from build123d import *
from build123d.topology import SkipClean

# Parameters (mm, degrees)
BOSS_EXTRUDE1_DEPTH  = 2
SKETCH12_R           = 25
BOSS_EXTRUDE2_DEPTH  = 8
CUT_EXTRUDE6_START   = -36
SKETCH17_R           = 10.33
CUT_EXTRUDE6_DEPTH   = 45.856111051
SKETCH25_R           = 30
BOSS_EXTRUDE3_DEPTH  = 5
CUT_EXTRUDE9_START   = -5
SKETCH26_R           = 10.33
CUT_EXTRUDE9_DEPTH   = 5
CUT_EXTRUDE10_DEPTH  = 45
FILLET3_R            = 1.5
MIRROR9_COPY_1_DEPTH = 45
FILLET3_OF_MIRROR9_R = 1.5
SKETCH29_R           = 10.33
CUT_EXTRUDE11_DEPTH  = 5


with BuildPart() as part:
    # Sketch3 → Boss-Extrude1 (new body)
    with BuildSketch(Plane(origin=(0, 0, 0), x_dir=(1, 0, 0), z_dir=(0, 1, 0))):
        Polygon((35.1, 0), (24.81944802, 24.81944802), (0, 35.1), (-24.81944802, 24.81944802), (-35.1, 0), (-24.81944802, -24.81944802), (0, -35.1), (24.81944802, -24.81944802), align=None)
    boss_extrude1 = extrude(amount=BOSS_EXTRUDE1_DEPTH)

    # Sketch12 → Boss-Extrude2 (add)
    with BuildSketch(Plane(origin=(0, 2, 0), x_dir=(1, 0, 0), z_dir=(0, 1, 0))):
        with Locations(Location((0, 0, 0), (0, 0, 270))):
            Circle(SKETCH12_R)
    boss_extrude2 = extrude(amount=BOSS_EXTRUDE2_DEPTH)

    # Sketch17 → Cut-Extrude6 (cut)
    with BuildSketch(Plane(origin=(0, 10, 0), x_dir=(1, 0, 0), z_dir=(0, 1, 0)).offset(CUT_EXTRUDE6_START)):
        with Locations(Location((0, 17, 0), (0, 0, 40.756206315))):
            Circle(SKETCH17_R)
    cut_extrude6 = extrude(amount=CUT_EXTRUDE6_DEPTH, mode=Mode.SUBTRACT)

    # Sketch25 → Boss-Extrude3 (add)
    with BuildSketch(Plane(origin=(0, 10, 0), x_dir=(1, 0, 0), z_dir=(0, 1, 0))):
        with Locations(Location((0, 0, 0), (0, 0, 270))):
            Circle(SKETCH25_R)
    boss_extrude3 = extrude(amount=BOSS_EXTRUDE3_DEPTH)

    # Sketch26 → Cut-Extrude9 (cut)
    with BuildSketch(Plane(origin=(0, 15, 0), x_dir=(1, 0, 0), z_dir=(0, 1, 0)).offset(CUT_EXTRUDE9_START)):
        with Locations(Location((0, 17, 0), (0, 0, 270))):
            Circle(SKETCH26_R)
    extrude(amount=CUT_EXTRUDE9_DEPTH, mode=Mode.SUBTRACT)

    # Sketch27 → Cut-Extrude10 (cut)
    with BuildSketch(Plane(origin=(0, 15, 0), x_dir=(1, 0, 0), z_dir=(0, 1, 0))):
        with BuildLine():
            Line((0, -20), (0, 4.5))
            ThreePointArc((0, 4.5), (-10.662403413, 8.877487957), (-21.5, 4.953746429))
            Line((-21.5, 4.953746429), (-21.5, -20))
            ThreePointArc((-21.5, -20), (-10.75, -24.149367106), (0, -20))
        make_face()
    cut_extrude10 = extrude(amount=-CUT_EXTRUDE10_DEPTH, mode=Mode.SUBTRACT)

    # Mirror8: Cut-Extrude10 across plane
    add(cut_extrude10.mirror(Plane.ZY), mode=Mode.SUBTRACT)

    # Fillet3
    fillet3_edges = [part.edges().sort_by_distance(p)[0] for p in [
        (12.40972401, 2, -29.95972401),
        (-12.40972401, 2, -29.95972401),
        (-29.95972401, 2, -12.40972401),
        (-29.95972401, 2, 12.40972401),
        (-12.40972401, 2, 29.95972401),
        (12.40972401, 2, 29.95972401),
        (29.95972401, 2, 12.40972401),
        (29.95972401, 2, -12.40972401),
    ]]
    fillet(fillet3_edges, radius=FILLET3_R)

    # Mirror9: Boss-Extrude1, Boss-Extrude2, Cut-Extrude6, Boss-Extrude3, Cut-Extrude10 across plane
    with SkipClean():  # the faces are left unmerged after this step: merging them gives an invalid solid
        add(boss_extrude1.mirror(Plane.ZX))
        add(boss_extrude2.mirror(Plane.ZX))
        add(cut_extrude6.mirror(Plane.ZX), mode=Mode.SUBTRACT)
        add(boss_extrude3.mirror(Plane.ZX))
        add(cut_extrude10.mirror(Plane.ZX), mode=Mode.SUBTRACT)

    # Mirror9 copy 1 sketch → Mirror9 copy 1 (cut)
    with SkipClean():  # the faces are left unmerged after this step: merging them gives an invalid solid
        with BuildSketch(Plane(origin=(0, -15, 0), x_dir=(-1, 0, 0), z_dir=(0, -1, 0))):
            with BuildLine():
                Line((0, -20), (0, 4.5))
                ThreePointArc((0, 4.5), (-10.662403413, 8.877487957), (-21.5, 4.953746429))
                Line((-21.5, 4.953746429), (-21.5, -20))
                ThreePointArc((-21.5, -20), (-10.75, -24.149367106), (0, -20))
            make_face()
        extrude(amount=-MIRROR9_COPY_1_DEPTH, mode=Mode.SUBTRACT)

    # Fillet3 of Mirror9
    fillet3_of_mirror9_edges = [part.edges().sort_by_distance(p)[0] for p in [
        (12.40972401, -2, -29.95972401),
        (-12.40972401, -2, -29.95972401),
        (-29.95972401, -2, -12.40972401),
        (-29.95972401, -2, 12.40972401),
        (-12.40972401, -2, 29.95972401),
        (12.40972401, -2, 29.95972401),
        (29.95972401, -2, 12.40972401),
        (29.95972401, -2, -12.40972401),
    ]]
    fillet(fillet3_of_mirror9_edges, radius=FILLET3_OF_MIRROR9_R)

    # Sketch29 → Cut-Extrude11 (cut)
    with SkipClean():  # the faces are left unmerged after this step: merging them gives an invalid solid
        with BuildSketch(Plane.XZ.offset(15)):
            with Locations(Location((0, -17, 0), (0, 0, 270))):
                Circle(SKETCH29_R)
        extrude(amount=-CUT_EXTRUDE11_DEPTH, mode=Mode.SUBTRACT)


solid = part.part
The listing builds one solid part. Answer for the finished solid, in the listing's coordinates (mm). A direction names the side the tool comes from. Give positions to 0.01 mm unless a question says otherwise; leave off trailing zeros. Loops run counter-clockwise (first coordinate to the right, second up) from the corner with the lowest first, then second, coordinate; pieces in that order, holes last.
Item 1: A cutting plane is placed at A-A (y = 5.25). Give the vertices of the cut face in (x, z), then the cut area to 3 significant figures.
Derived:
outline: (-21.5, -4.95) - (-21.5, 12.76) arc R25 ccw to (-7.82, -23.74) arc R10.33 cw (long way) to (7.82, -23.74) arc R25 ccw to (21.5, 12.76) - (21.5, -4.95) arc R16 cw to (0, -4.5) arc R16 cw to start; (-7.56, 23.83) arc R16 cw to (0, 20) arc R16 cw to (7.56, 23.83) arc R25 ccw to start
area: 441 mm2
Item 2: Each of these flat-tipped pins is pushed along its axis until it touches: pin 1 Ø1 at (x, y) = (9, -5.5) entering from -Z; pin 2 Ø3 at (y, z) = (0, -10) entering from -X; pin 3 Ø10 at (y, z) = (-5, -14.5) entering from +X; pin 4 Ø12.5 at (x, z) = (0, -17) entering from +Y. Where does it stop, or does it pass through?
Derived:
pin 1: stops at z = -23.51
pin 2: stops at x = -31.58
pin 3: stops at x = 30.26
pin 4: passes through
Item 3: Find the intervals of material crossed by line 1 along Y through (x, z) = (-24.5, 17); line 2 along Z through (x, y) = (0, -3.5); line 3 along X through (y, z) = (10.75, 21), in increasing order.
Derived:
line 1: y = -15 to -10, -2 to 2, 10 to 15
line 2: z = -6.67 to -4.5, 20 to 25
line 3: x = -21.42 to -20.28, -1.22 to 1.22, 20.28 to 21.42
Item 4: A cutting plane is placed at B-B (y = 11.5). Give the vertices of the cut face in (x, z), then the cut area to 3 significant figures.
Derived:
outline: circle Ø60 at (0, 0); hole (-21.5, -4.95) arc R16 ccw to (0, -4.5) arc R16 ccw to (21.5, -4.95) - (21.5, 20) arc R16 ccw to (0, 20) arc R16 ccw to (-21.5, 20) - close; hole circle Ø20.66 at (0, -17)
area: 1,180 mm2
Item 5: A tool of negligible diameter and unlimited length cuts with its end or side. For faces 5 (the flat face through (-15.4, -10, -20.1)), 6 (the cylindrical face through (-8.305, -0.21, 23.961)), 7 (the cylindrical face through (1.32, 12.46, -29.97)), from which of +Z, -Z, +X, -X, +Y, -Y can it reach the whole face along a straight path? Write none if from no direction.
Derived:
face 5: none
face 6: +Y, -Y
face 7: +Y
Item 6: A cutting plane is placed at C-C (x = -15). Give the number of separate pieces and of enclosed holes in the cut face, then the cut area to 3 significant figures.
Derived:
separate pieces: 4
enclosed holes: 0
area: 487 mm2
Item 7: Determine the mould class of faces 1 (the cylindrical face through (1.32, -12.46, -29.97)), 2 (the cylindrical face through (0, -6, 25)), 3 (the cylindrical face through (-29.615, -1.572, -12.063)), 4 (the flat face through (9, 15, -9)) for opening direction Y: +Y half, -Y half, draft (parallel to the pull), parting line (faces both ways), or undercut.
Derived:
face 1: draft
face 2: undercut
face 3: -Y half
face 4: +Y half
